The model under review builds one solid part; all positions refer to its coordinate system, in mm. A direction names the side the tool comes from. Round coordinates to 2 decimals unless told otherwise and drop trailing zeros. Order: outer loops, then holes, each group sorted by start corner. A loop starts at its lowest first (then second) coordinate and runs counter-clockwise, first axis right, second up. Notation, with made-up numbers: (70.5, 14) -> (76.5, 14) arc R17 cw to (76.5, 25) -> close; hole circle Ø1 at (24.25, 68.25). An arc over 180 degrees is marked (long way). Return JSON: item names as keys, results as strings. Group by question number.
from build123d import *

# Parameters (mm, degrees)
SKETCH1_R              = 1.55
BOSS_EXTRUDE1_DEPTH    = 33
CUT_EXTRUDE2_START     = 3
CUT_EXTRUDE2_OUTLINE_R = 1.55
CUT_EXTRUDE2_DEPTH     = 30
BOSS_EXTRUDE3_START    = 15.4
SKETCH7_R              = 1.6
BOSS_EXTRUDE3_DEPTH    = 11
SKETCH14_R             = 1.6
BOSS_EXTRUDE4_DEPTH    = 9


# Read off the part's stored shape, not the designer's step: Cut-Extrude2
with BuildPart() as part:
    # Sketch1 → Boss-Extrude1 (new body)
    with BuildSketch(Plane.XY):
        with BuildLine():
            Line((9.5, 1.5), (9.5, 1.25))
            ThreePointArc((9.5, 1.25), (9.133883476, 0.366116524), (8.25, 0))
            Line((8.25, 0), (4.242640687, 0))
            ThreePointArc((4.242640687, 0), (3.09459039, 0.228361402), (2.121320344, 0.878679656))
            Line((2.121320344, 0.878679656), (0.878679656, 2.121320344))
            ThreePointArc((0.878679656, 2.121320344), (0.228361402, 3.09459039), (0, 4.242640687))
            Line((0, 4.242640687), (0, 8.25))
            ThreePointArc((0, 8.25), (0.366116524, 9.133883476), (1.25, 9.5))
            Line((1.25, 9.5), (1.5, 9.5))
            Line((1.5, 9.5), (1.5, 5))
            Line((1.5, 5), (3.5, 5))
            Line((3.5, 5), (3.5, 11))
            Line((3.5, 11), (8.5, 11))
            ThreePointArc((8.5, 11), (10.267766953, 10.267766953), (11, 8.5))
            Line((11, 8.5), (11, 3.5))
            Line((11, 3.5), (5, 3.5))
            Line((5, 3.5), (5, 1.5))
            Line((5, 1.5), (9.5, 1.5))
        make_face()
        with Locations((8.5, 8.5)):
            Circle(SKETCH1_R, mode=Mode.SUBTRACT)
    extrude(amount=BOSS_EXTRUDE1_DEPTH)

    # Cut-Extrude2 outline → Cut-Extrude2 (cut)
    with BuildSketch(Plane.XY.offset(CUT_EXTRUDE2_START)):
        with BuildLine():
            Line((3.5, 8.5), (4, 8.5))
            ThreePointArc((4, 8.5), (5.318019485, 5.318019485), (8.5, 4))
            Line((8.5, 4), (8.5, 3.5))
            Line((8.5, 3.5), (11, 3.5))
            Line((11, 3.5), (11, 8.5))
            ThreePointArc((11, 8.5), (10.267766953, 10.267766953), (8.5, 11))
            Line((8.5, 11), (3.5, 11))
            Line((3.5, 11), (3.5, 8.5))
        make_face()
        with Locations((8.5, 8.5)):
            Circle(CUT_EXTRUDE2_OUTLINE_R, mode=Mode.SUBTRACT)
    extrude(amount=CUT_EXTRUDE2_DEPTH, mode=Mode.SUBTRACT)

    # Sketch7 → Boss-Extrude3 (add)
    with BuildSketch(Plane.XY.offset(BOSS_EXTRUDE3_START)):
        with BuildLine():
            Line((8.5, 6), (8.5, 4))
            ThreePointArc((8.5, 4), (5.318019485, 5.318019485), (4, 8.5))
            Line((4, 8.5), (6, 8.5))
            ThreePointArc((6, 8.5), (10.267766953, 10.267766953), (8.5, 6))
        make_face()
        with Locations((8.5, 8.5)):
            Circle(SKETCH7_R, mode=Mode.SUBTRACT)
    extrude(amount=BOSS_EXTRUDE3_DEPTH)

    # Sketch14 → Boss-Extrude4 (add)
    with BuildSketch(Plane.XY.offset(4.7)):
        with BuildLine():
            Line((6, 8.5), (4, 8.5))
            ThreePointArc((4, 8.5), (5.318019485, 5.318019485), (8.5, 4))
            Line((8.5, 4), (8.5, 6))
            ThreePointArc((8.5, 6), (10.267766953, 10.267766953), (6, 8.5))
        make_face()
        with Locations((8.5, 8.5)):
            Circle(SKETCH14_R, mode=Mode.SUBTRACT)
    extrude(amount=BOSS_EXTRUDE4_DEPTH)


solid = part.part
Item 1: Consider section D-D on x = 6.5. State the section outline as (y, z) points, plus the area to 3 significant figures.
Item 2: Consider section C-C on y = 9. State the section outline as (x, z) points.
Item 3: The part is to be moulded in two halves that separate along X. For faces 4 (the face through (5.283, 5.353, 29.654)), 5 (the face through (7.23, 7.53, 9.14)), 6 (the face through (6.8, 7.5, 26.4)), say which applies: +X half, -X half, draft (parallel to the pull), parting line (faces both ways), or undercut.
Item 4: Insertion check: pin 1 Ø2 at (x, y) = (7.5, 8.5) entering from +Z; pin 2 Ø0.6 at (x, z) = (3, 9) entering from +Y; pin 3 Ø0.8 at (y, z) = (5, 10.5) entering from +X. Each pin has a flat end and moves straight along its axis. Give the tip position at first contact, or say it passes through.
Item 5: Consider section A-A on z = 10. State the section outline as (x, y) points, plus the area to 3 significant figures.
Item 6: For faces 1 (the face through (5.283, 5.353, 14.538)), 2 (the face through (10.325, 10.209, 9.137)), 3 (the face through (3.5, 7, 16)), list the 3-axis set-ups (+Z, -Z, +X, -X, +Y, -Y) from which the entire face can be reached by the end or side of a thin tool; tool diameter is ignored.
Item 7: Consider section B-B on z = 14. State the section outline as (x, y) points.
Item 8: Wall thickness on line 1 along Z through (x, y) = (5.25, 5.5); line 2 along Y through (x, z) = (8.5, 1.7); line 3 along X through (y, z) = (8, 6.5): over which ranges is each line inside the solid? List them lowest first.
Values:
{
 "1": {"outline": "(0, 0) -> (1.5, 0) -> (1.5, 33) -> (0, 33) -> close; (3.5, 0) -> (11, 0) -> (11, 3) -> (4.47, 3) -> (4.47, 4.7) -> (10, 4.7) -> (10, 13.7) -> (4.47, 13.7) -> (4.47, 15.4) -> (10, 15.4) -> (10, 26.4) -> (4.47, 26.4) -> (4.47, 33) -> (3.5, 33) -> close", "area": "212 mm^2"},
 "2": {"outline": "(0.25, 0) -> (1.5, 0) -> (1.5, 33) -> (0.25, 33) -> close; (3.5, 0) -> (7.03, 0) -> (7.03, 3) -> (3.5, 3) -> close; (6.05, 4.7) -> (6.98, 4.7) -> (6.98, 13.7) -> (6.05, 13.7) -> close; (6.05, 15.4) -> (6.98, 15.4) -> (6.98, 26.4) -> (6.05, 26.4) -> close; (9.97, 0) -> (10.95, 0) -> (10.95, 3) -> (9.97, 3) -> close; (10.02, 4.7) -> (10.95, 4.7) -> (10.95, 13.7) -> (10.02, 13.7) -> close; (10.02, 15.4) -> (10.95, 15.4) -> (10.95, 26.4) -> (10.02, 26.4) -> close"},
 "3": {"face 4": "+X half", "face 5": "undercut", "face 6": "draft"},
 "4": {"pin 1": "z = 26.4", "pin 2": "y = 5", "pin 3": "x = 8.5"},
 "5": {"outline": "(0, 4.24) arc R3 ccw to (0.88, 2.12) -> (2.12, 0.88) arc R3 ccw to (4.24, 0) -> (8.25, 0) arc R1.25 ccw to (9.5, 1.25) -> (9.5, 1.5) -> (5, 1.5) -> (5, 3.5) -> (8.5, 3.5) -> (8.5, 6) arc R2.5 ccw (long way) to (6, 8.5) -> (3.5, 8.5) -> (3.5, 5) -> (1.5, 5) -> (1.5, 9.5) -> (1.25, 9.5) arc R1.25 ccw to (0, 8.25) -> close; hole circle Ø3.2 at (8.5, 8.5)", "area": "62.4 mm^2"},
 "6": {"face 1": "+X, +Y", "face 2": "+Z", "face 3": "+Z, -Z, +Y"},
 "7": {"outline": "(0, 4.24) arc R3 ccw to (0.88, 2.12) -> (2.12, 0.88) arc R3 ccw to (4.24, 0) -> (8.25, 0) arc R1.25 ccw to (9.5, 1.25) -> (9.5, 1.5) -> (5, 1.5) -> (5, 3.5) -> (8.5, 3.5) -> (8.5, 4) arc R4.5 cw to (4, 8.5) -> (3.5, 8.5) -> (3.5, 5) -> (1.5, 5) -> (1.5, 9.5) -> (1.25, 9.5) arc R1.25 ccw to (0, 8.25) -> close"},
 "8": {"line 1": "0 to 3, 4.7 to 13.7, 15.4 to 26.4", "line 2": "0.03 to 1.5, 3.5 to 6.95, 10.05 to 11", "line 3": "0 to 1.5, 3.5 to 6.98, 10.02 to 10.95"}
}
